from build123d import *

# Parameters (mm, degrees)
ESQUISSE1_W        = 20
ESQUISSE1_H        = 20
BOSS_EXTRU_1_DEPTH = 5
CHANFREIN1_SIZE    = 1


with BuildPart() as part:
    # Esquisse1 → Boss.-Extru.1 (new body)
    with BuildSketch(Plane.XY):
        with Locations((10, -10)):
            Rectangle(ESQUISSE1_W, ESQUISSE1_H)
    extrude(amount=BOSS_EXTRU_1_DEPTH)

    # Chanfrein1
    chanfrein1_edges = [part.edges().sort_by_distance(p)[0] for p in [
        (20, -10, 5),
        (10, 0, 5),
        (0, -10, 5),
        (10, -20, 5),
    ]]
    chamfer(chanfrein1_edges, length=CHANFREIN1_SIZE)


solid = part.part
For this review, take the finished solid that the model builds, in its own axes (mm). Round coordinates to 2 decimals unless told otherwise and drop trailing zeros. Loops run counter-clockwise (first coordinate to the right, second up) from the corner with the lowest first, then second, coordinate; pieces in that order, holes last. Notation, with made-up numbers: (39.5, -29.5) - (88.5, -29.5) arc R21 ccw to (88.5, 0.5) - close; hole circle Ø4 at (-22.5, 2.5). An arc over 180 degrees is marked (long way). One line per item, written item: value. Start each with the question number.
Item 1: For L1, parallel to Y at x = 15.25, z = 4.65; L2, parallel to Y at x = 3.5, z = 4.5; L3, parallel to Z at x = 11.75, y = -0.75, list the stretches that pass through material, from the lowest coordinate up.
Item 2: Take a section at A-A (z = 4.35). Give the boundary of the cut face in (x, y), plus the area to 3 significant figures.
Item 3: Clearance check with a flat-ended pin moving along its axis: pin 1 Ø3 at (x, y) = (5, -11) entering from -Z. State where the tip first meets the part, or that it passes through.
Answer below:
1. L1: y = -19.35 to -0.65
1. L2: y = -19.5 to -0.5
1. L3: z = 0 to 4.75
2. outline: (0.35, -19.65) - (19.65, -19.65) - (19.65, -0.35) - (0.35, -0.35) - close
2. area: 372 mm2
3. pin 1: stops at z = 0
